Part model, mm, in its own coordinate system. A direction names the side the tool comes from. Coordinates: 2 decimals unless noted, no trailing zeros. Write each loop counter-clockwise with the first axis right and the second up, starting at its lowest first coordinate (ties: lowest second). Pieces come first, ordered by that corner, then holes. Notation, with made-up numbers: (16.5, 84.5) - (62.5, 84.5) arc R31 ccw to (62.5, 121.5) - close; hole circle Ø3 at (31, 49). An arc over 180 degrees is marked (long way). Write each question's results on one line, items separated by ' | '.
from build123d import *

# Parameters (mm, degrees)
F0_R     = 2.5
F0_R_2   = 3.5
F1_DEPTH = 3
F2_SIZE  = 2
F4_R     = 0.5
F5_DEPTH = 2
F5_TAPER = 45


# Not quite as in the source:
# - a pattern or mirror of a feature is missing from the dataset's text; its kind, count and spacing are read off the source's solid


with BuildPart() as f1:
    # F0 (on Top) → F1 (new body, symmetric)
    with BuildSketch(Plane.XY):
        with BuildLine():
            Line((-22.6589401231, 2.4236629568), (-39.5600539291, 2.4236629568))
            Line((-39.5600539291, 2.4236629568), (-39.5600539291, -7.3263370432))
            Line((-39.5600539291, -7.3263370432), (-31.8100539291, -7.3263370432))
            ThreePointArc((-31.8100539291, -7.3263370432), (-7.74599031, -5.7290436956), (15.4584982429, -12.300361288))
            Line((15.4584982429, -12.300361288), (29.0535219773, -13.773592777))
            Line((29.0535219773, -13.773592777), (33.4806282794, -13.7333460718))
            ThreePointArc((33.4806282794, -13.7333460718), (38.7220078669, -10.5438462203), (42.4399460709, -5.663077347))
            ThreePointArc((42.4399460709, -5.663077347), (43.0076744864, -4.0355880404), (41.3801851798, -3.4678596249))
            Line((41.3801851798, -3.4678596249), (39.4420786101, -4.4034978191))
            Line((39.4420786101, -4.4034978191), (36.8522457248, -5.3948726996))
            Line((36.8522457248, -5.3948726996), (31.776658302, -4.1156165412))
            ThreePointArc((31.776658302, -4.1156165412), (22.9700739727, -0.8151163334), (15.0904607998, 4.3191728497))
            ThreePointArc((15.0904607998, 4.3191728497), (8.5263135264, 7.5598223627), (1.2061465951, 7.6304961974))
            Line((1.2061465951, 7.6304961974), (-22.6589401231, 2.4236629568))
        make_face()
        with Locations((-34.5600539291, -2.8220066844)):
            Circle(F0_R, mode=Mode.SUBTRACT)
        with Locations((4.4399460709, 0)):
            Circle(F0_R_2, mode=Mode.SUBTRACT)
    extrude(amount=F1_DEPTH, both=True)

    # F2
    f2_edges = [f1.edges().sort_by_distance(p)[0] for p in [
        (22.25601, -13.036977, 3),
        (22.25601, -13.036977, -3),
        (31.267075, -13.753469, 3),
        (31.267075, -13.753469, -3),
        (38.722008, -10.543846, 3),
        (38.722008, -10.543846, -3),
    ]]
    chamfer(f2_edges, length=F2_SIZE)

    # F4
    f4_edges = [f1.edges().sort_by_distance(p)[0] for p in [
        (0.939946, 0, -3),
        (-37.060054, -2.822007, -3),
        (-37.060054, -2.822007, 3),
        (0.939946, 0, 3),
    ]]
    fillet(f4_edges, radius=F4_R)

    # F3 (on face) → F5 (cut)
    with BuildSketch(Plane(origin=(0, 0, -3), x_dir=(1, 0, 0), z_dir=(0, 0, -1))):
        Polygon((11.9156481301, 15.2815678021), (9.0032261915, 9.5891237242), (21.4353172765, 0), (52.8852939606, 0), (52.8852939606, 15.2815678021), align=None)
    f5 = extrude(amount=-F5_DEPTH, taper=F5_TAPER, mode=Mode.SUBTRACT)

    # F5_copies: F5 across plane
    add(f5.mirror(Plane.XY), mode=Mode.SUBTRACT)


solid = f1.part
(1) Flat gauge pins, fed straight in: P1, Ø5.5, axis at x = 25.5, y = -10, coming from the +Z side; P2, Ø2, axis at x = -12.5, z = 0.5, coming from the -Y side; P3, Ø1, axis at x = 9.5, z = 0.5, coming from the -Y side. Where does each tip first touch, or does it go through?
Return value:
P1: stops at z = 1 | P2: stops at y = -5.43 | P3: stops at y = -9.96
(2) Saw through at C-C on y = 5.75. Write the cut outline in (x, z), then the cut area to 3 significant figures.
Return value:
outline: (-7.41, -3) - (13.03, -3) - (13.03, 3) - (-7.41, 3) - close | area: 123 mm^2
(3) Saw through at B-B on x = -25. Write the cut outline in (y, z), then the cut area to 3 significant figures.
Return value:
outline: (-6.03, -3) - (2.42, -3) - (2.42, 3) - (-6.03, 3) - close | area: 50.7 mm^2
(4) Two-plate mould, pull along Y, no slides. Class faces 6 (the flat face through (-31, 2.424, 0)), 7 (the cylindrical face through (-32.25, -3.78, -0.04)), 8 (the flat face through (-9, -1, 3)): released by +Y, released by -Y, zero draft, split by the parting line, or undercut.
Return value:
face 6: released by +Y | face 7: undercut | face 8: zero draft
(5) Wall check: line 1 (X direction, y = -2.75, z = 1.5) (3 decimals); line 2 (X direction, y = -1.75, z = -1.5); line 3 (Z direction, x = 28.5, y = -9.5). Give the ranges that are in metal, low to high. Write a range as from..to.
Return value:
line 1: x = -39.56..-37.059, -32.061..2.275, 6.605..20.326 | line 2: x = -39.56..-36.82, -32.3..1.41, 7.47..21.62 | line 3: z = -1..1
(6) Saw through at A-A on z = 0. Write the cut outline in (x, y), then the cut area to 3 significant figures.
Return value:
outline: (-39.56, -7.33) - (-31.81, -7.33) arc R70.81 cw to (15.46, -12.3) - (29.05, -13.77) - (33.48, -13.73) arc R16.54 ccw to (42.44, -5.66) arc R1.22 ccw to (41.38, -3.47) - (39.44, -4.4) - (36.85, -5.39) - (31.78, -4.12) arc R43.05 cw to (15.09, 4.32) arc R16.44 ccw to (1.21, 7.63) - (-22.66, 2.42) - (-39.56, 2.42) - close; hole circle Ø5 at (-34.56, -2.82); hole circle Ø7 at (4.44, 0) | area: 867 mm^2
(7) 3-axis set-ups, long thin cutter, end or side, ignore diameter. For faces 1 (the flat face through (22.161, -13.027, 0.014)), 2 (the flat face through (27, -8, 1)), 3 (the flat face through (27, -8, -1)), 4 (the flat face through (34.35, -4.764, 0.014)), 5 (the flat face through (-9, -1, -3)): which of +Z, -Z, +X, -X, +Y, -Y reach the whole face in a straight line?
Return value:
face 1: +Z, -Z, -X, -Y | face 2: +Z, +X | face 3: -Z, +X | face 4: +Z, -Z, +Y | face 5: -Z, +X, -X, +Y, -Y
